Source: CAD feature listing. Evaluate the final solid. Frame: model axes, mm. Face numbers are marked on the shaded views. A direction names the side the tool comes from. Round coordinates to 2 decimals unless told otherwise and drop trailing zeros. Loops run counter-clockwise (first coordinate to the right, second up) from the corner with the lowest first, then second, coordinate; pieces in that order, holes last. Notation, with made-up numbers: (45.5, 88.25) - (99.5, 88.25) arc R10 cw to (99.5, 95.25) - close; hole circle Ø2 at (35, 85.5). An arc over 180 degrees is marked (long way). One line per question, with ' | ' between items.
from build123d import *

# Parameters (mm, degrees)
F0_W     = 35
F0_H     = 25
F1_DEPTH = 10
F3_T     = -1
F2_R     = 3
F2_R_2   = 2.5
F4_DEPTH = 3
F5_DEPTH = 1


with BuildPart() as f1:
    # F0 (on Top) → F1 (new body)
    with BuildSketch(Plane.XY):
        with Locations((-20.4494718197, 12.5)):
            Rectangle(F0_W, F0_H)
    extrude(amount=F1_DEPTH)

    # F3
    f3_openings = [f1.faces().sort_by_distance(p)[0] for p in [
        (-20.449472, 12.5, 10),
    ]]
    offset(amount=F3_T, openings=f3_openings)

    # F2 (on face) → F4 (join)
    with BuildSketch(Plane.XZ):
        with Locations((-29.2118718197, 5)):
            Circle(F2_R)
        with Locations((-29.2118718197, 5)):
            Circle(F2_R_2, mode=Mode.SUBTRACT)
        with Locations((-11.6870718197, 5)):
            Circle(F2_R)
        with Locations((-11.6870718197, 5)):
            Circle(F2_R_2, mode=Mode.SUBTRACT)
    extrude(amount=F4_DEPTH)

    # F5 (cut): faces of the model
    f5_faces = [f1.faces().sort_by_distance(p)[0] for p in [
        (-29.2118718197, 0, 5),
        (-11.6870718197, 0, 5),
    ]]
    extrude(f5_faces, amount=-F5_DEPTH, mode=Mode.SUBTRACT)


solid = f1.part
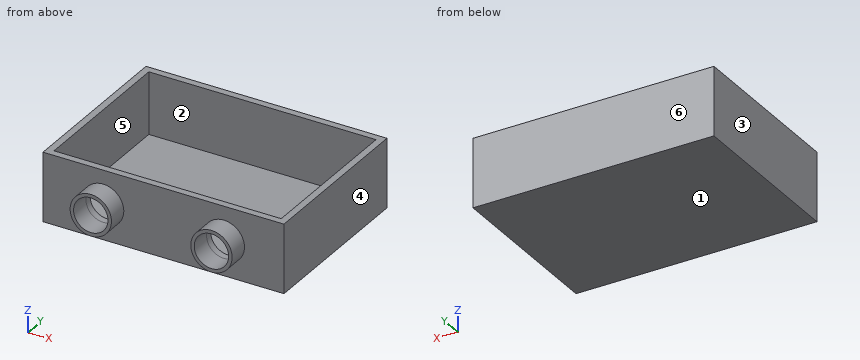
1. Contact query for flat-ended pins moving along their axis: P1, Ø8, axis at x = -29, y = 19.5, coming from the +Z side; P2, Ø4, axis at x = -29.21, z = 5, coming from the -Y side. Output: stop coordinate, or through.
Worked out:
P1: stops at z = 1 | P2: stops at y = 24
2. Section query A-A, the plane z = 5. Return loops of the section in (x, y).
Worked out:
outline: (-37.95, 0) - (-32.21, 0) - (-32.21, -3) - (-31.71, -3) - (-31.71, 1) - (-36.95, 1) - (-36.95, 24) - (-3.95, 24) - (-3.95, 1) - (-9.19, 1) - (-9.19, -3) - (-8.69, -3) - (-8.69, 0) - (-2.95, 0) - (-2.95, 25) - (-37.95, 25) - close; (-26.71, -3) - (-26.21, -3) - (-26.21, 0) - (-14.69, 0) - (-14.69, -3) - (-14.19, -3) - (-14.19, 1) - (-26.71, 1) - close
3. Section query C-C, the plane y = -0.5. Return loops of the section in (x, z).
Worked out:
outline: circle Ø6 at (-29.21, 5); circle Ø6 at (-11.69, 5); hole circle Ø5 at (-29.21, 5); hole circle Ø5 at (-11.69, 5)
4. Section query B-B, the plane z = 8.5. Return loops of the section in (x, y).
Worked out:
outline: (-37.95, 0) - (-2.95, 0) - (-2.95, 25) - (-37.95, 25) - close; hole (-36.95, 1) - (-3.95, 1) - (-3.95, 24) - (-36.95, 24) - close
5. Access query for the marked faces 1 and 2. Directions: +Z, -Z, +X, -X, +Y, -Y. A direction counts if a zero-diameter tool reaches every point of the face in a straight line with its end or side. Return the directions, or none.
Worked out:
face 1: -Z, +X, -X, +Y, -Y | face 2: +Z
6. Mould query, pull axis X, two halves, no side actions, for the marked faces 3, 4, 5 and 6. Classes: released by +X, released by -X, zero draft, split by the parting line, or undercut.
Worked out:
face 3: released by -X | face 4: released by +X | face 5: undercut | face 6: zero draft
7. Material intervals for probe 1 along X at (y, z) = (8, 3.75); probe 2 along Y at (x, z) = (-15.5, 4.5); probe 3 along Z at (x, y) = (-8, 18), sorted ascending.
Worked out:
probe 1: x = -37.95 to -36.95, -3.95 to -2.95 | probe 2: y = 0 to 1, 24 to 25 | probe 3: z = 0 to 1
8. Section query D-D, the plane y = 23.25. Return loops of the section in (x, z).
Worked out:
outline: (-37.95, 0) - (-2.95, 0) - (-2.95, 10) - (-3.95, 10) - (-3.95, 1) - (-36.95, 1) - (-36.95, 10) - (-37.95, 10) - close
